Here's the drawing with two shaded views (mm, measured from the low corner). I have some questions. Round coordinates to 2 decimals unless told otherwise and drop trailing zeros. Loops run counter-clockwise (first coordinate to the right, second up) from the corner with the lowest first, then second, coordinate; pieces in that order, holes last.
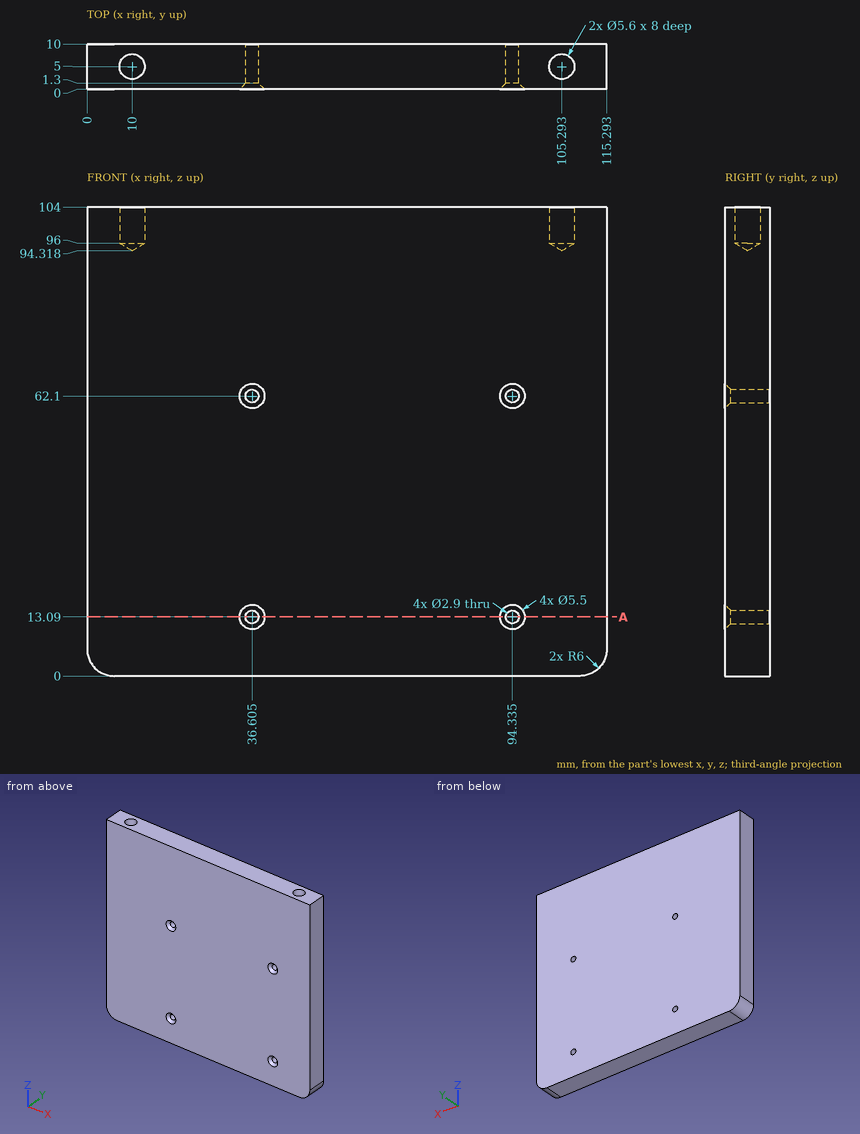
Item 1: Will these pins go through, and if not, where does the flat tip stop? pin 1 (1.7 mm diameter, centred on x = 94.335, z = 62.1, fed in from -Y); pin 2 (4 mm diameter, centred on x = 36.605, z = 13.09, fed in from -Y).
Results list:
pin 1: passes through
pin 2: stops at y = 0.75
Item 2: If we section it at A-A, the plane z = 13.09: Please give me the cut outline in (x, y) (1 decimal).
Results list:
outline: (0, 0) - (33.9, 0) - (35.2, 1.3) - (35.2, 10) - (0, 10) - close; (38.1, 1.3) - (39.4, 0) - (91.6, 0) - (92.9, 1.3) - (92.9, 10) - (38.1, 10) - close; (95.8, 1.3) - (97.1, 0) - (115.3, 0) - (115.3, 10) - (95.8, 10) - close
Item 3: If I drill on line 1 along X through (y, z) = (5, 99); line 2 along Z through (x, y) = (94, 7), over which ranges is the centre line in solid material (lowest first)?
Results list:
line 1: x = 0 to 7.2, 12.8 to 102.49, 108.09 to 115.29
line 2: z = 0 to 11.68, 14.5 to 60.69, 63.51 to 104
